Could you check a few things on this model? Use its own coordinates, in mm. Round coordinates to 2 decimals unless told otherwise and drop trailing zeros. Write each loop counter-clockwise with the first axis right and the second up, starting at its lowest first coordinate (ties: lowest second). Pieces come first, ordered by that corner, then holes. Notation, with made-up numbers: (63, 30.5) -> (108, 30.5) arc R18 cw to (108, 46.5) -> close; hole circle Ø9 at (-38.75, 48.25). An arc over 180 degrees is marked (long way). Return JSON: item names as keys, results as strings.
from build123d import *

# Parameters (mm, degrees)
SKETCH1_R         = 88
HUB_DEPTH         = 40
SKETCH2_R         = 4
BORE_DEPTH        = 40
SKETCH3_R         = 1.25
CLAMP_SCREW_DEPTH = 85


with BuildPart() as part:
    # Sketch1 → Hub (new body)
    with BuildSketch(Plane.XY):
        Circle(SKETCH1_R)
    extrude(amount=HUB_DEPTH)

    # Sketch2 → Bore (cut)
    with BuildSketch(Plane.XY):
        Circle(SKETCH2_R)
    extrude(amount=BORE_DEPTH, mode=Mode.SUBTRACT)

    # Sketch3 → Clamp_screw (cut)
    with BuildSketch(Plane(origin=(3.5, 0, 0), x_dir=(0, 0, -1), z_dir=(1, 0, 0))):
        with Locations(Location((-20, 0, 0), (0, 0, 180))):
            Circle(SKETCH3_R)
    extrude(amount=CLAMP_SCREW_DEPTH, mode=Mode.SUBTRACT)


solid = part.part
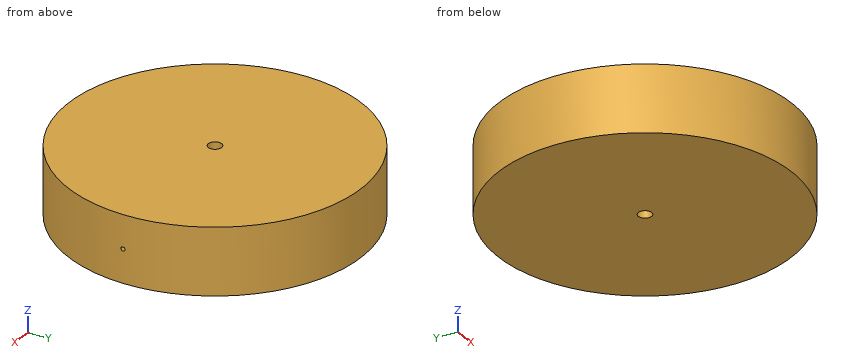
1) I want a section at B-B, the plane z = 3.5. Please give me the cut outline in (x, y).
Return value:
{"outline": "circle Ø176 at (0, 0); hole circle Ø8 at (0, 0)"}
2) I want a section at A-A, the plane x = 0. Please give me the cut outline in (y, z), and give its area (3 significant figures).
Return value:
{"outline": "(-88, 0) -> (-4, 0) -> (-4, 40) -> (-88, 40) -> close; (4, 0) -> (88, 0) -> (88, 40) -> (4, 40) -> close", "area": "6,720 mm²"}
3) If I drill on probe 1 along Y at (x, z) = (0, 26); probe 2 along Y at (x, z) = (3.5, 36); probe 3 along X at (y, z) = (12.5, 33), over which ranges is the centre line in solid material (lowest first)? Write a range as [from, to].
Return value:
{"probe 1": "[-88, -4], [4, 88]", "probe 2": "[-87.93, -1.94], [1.94, 87.93]", "probe 3": "[-87.11, 87.11]"}
4) I want a section at D-D, the plane y = -36. Please give me the cut outline in (x, z), and give its area (3 significant figures).
Return value:
{"outline": "(-80.3, 0) -> (80.3, 0) -> (80.3, 40) -> (-80.3, 40) -> close", "area": "6,420 mm²"}
5) I want a section at C-C, the plane x = 59. Please give me the cut outline in (y, z), and give its area (3 significant figures).
Return value:
{"outline": "(-65.29, 0) -> (65.29, 0) -> (65.29, 40) -> (-65.29, 40) -> close; hole circle Ø2.5 at (0, 20)", "area": "5,220 mm²"}
6) Will these pins go through, and if not, where does the flat tip stop? pin 1 Ø5 at (x, z) = (-51.5, 8.5) entering from -Y; pin 2 Ø4 at (x, z) = (-4.5, 19.5) entering from -Y; pin 3 Ø12 at (x, z) = (61, 27) entering from +Y (3 decimals); pin 4 Ø5 at (x, y) = (0, 0) entering from +Z.
Return value:
{"pin 1": "y = -73.1", "pin 2": "y = -87.96", "pin 3": "y = 68.695", "pin 4": "through"}
